from build123d import *

# Parameters (mm, degrees)
SKETCH1_W           = 60
SKETCH1_H           = 80
BOSS_EXTRUDE1_DEPTH = 4
SKETCH2_R           = 1.25
CUT_EXTRUDE1_DEPTH  = 51.159744816
BOSS_EXTRUDE2_START = 2
SKETCH3_R           = 3
SKETCH3_R_2         = 1.25
BOSS_EXTRUDE2_DEPTH = 2
SKETCH4_R           = 1.25
CUT_EXTRUDE2_DEPTH  = 51.358713248
BOSS_EXTRUDE3_START = 2
SKETCH5_R           = 3
SKETCH5_R_2         = 1.25
BOSS_EXTRUDE3_DEPTH = 2
SKETCH7_W           = 12.5
SKETCH7_H           = 12.5
CUT_EXTRUDE4_DEPTH  = 4
FILLET3_R           = 1
FILLET2_R           = 3
SKETCH8_W           = 60
SKETCH8_H           = 9
BOSS_EXTRUDE4_DEPTH = 7
CHAMFER1_SIZE       = 2
SKETCH9_R           = 1.45
CUT_EXTRUDE5_DEPTH  = 8


with BuildPart() as part:
    # Sketch1 → Boss-Extrude1 (new body)
    with BuildSketch(Plane.XY):
        Rectangle(SKETCH1_W, SKETCH1_H)
    extrude(amount=BOSS_EXTRUDE1_DEPTH)

    # Sketch2 → Cut-Extrude1 (cut, through all)
    with BuildSketch(Plane.XY.offset(4)):
        with Locations((-24.5, 25)):
            Circle(SKETCH2_R)
        with Locations(Location((24.5, 25, 0), (0, 0, 180))):
            Circle(SKETCH2_R)
        with Locations((24.5, -33)):
            Circle(SKETCH2_R)
        with Locations(Location((-24.5, -33, 0), (0, 0, 180))):
            Circle(SKETCH2_R)
    extrude(amount=-CUT_EXTRUDE1_DEPTH, mode=Mode.SUBTRACT)

    # Sketch3 → Boss-Extrude2 (add)
    # profile 1 of 4: a face of its own
    with BuildSketch(Plane.XY.offset(4).offset(BOSS_EXTRUDE2_START)):
        with Locations((-24.5, 25)):
            Circle(SKETCH3_R)
        with Locations((-24.5, 25)):
            Circle(SKETCH3_R_2, mode=Mode.SUBTRACT)
    # profile 2 of 4: a face of its own
    with BuildSketch(Plane.XY.offset(4).offset(BOSS_EXTRUDE2_START)):
        with Locations((24.5, 25)):
            Circle(SKETCH3_R)
        with Locations((24.5, 25)):
            Circle(SKETCH3_R_2, mode=Mode.SUBTRACT)
    # profile 3 of 4: a face of its own
    with BuildSketch(Plane.XY.offset(4).offset(BOSS_EXTRUDE2_START)):
        with Locations((24.5, -33)):
            Circle(SKETCH3_R)
        with Locations((24.5, -33)):
            Circle(SKETCH3_R_2, mode=Mode.SUBTRACT)
    # profile 4 of 4: a face of its own
    with BuildSketch(Plane.XY.offset(4).offset(BOSS_EXTRUDE2_START)):
        with Locations((-24.5, -33)):
            Circle(SKETCH3_R)
        with Locations((-24.5, -33)):
            Circle(SKETCH3_R_2, mode=Mode.SUBTRACT)
    extrude(amount=-BOSS_EXTRUDE2_DEPTH)

    # Sketch4 → Cut-Extrude2 (cut, through all)
    with BuildSketch(Plane(origin=(0, 0, 0), x_dir=(-1, 0, 0), z_dir=(0, 0, -1))):
        with Locations((-18.772703202, -17.1)):
            Circle(SKETCH4_R)
        with Locations((9.127296798, -17.1)):
            Circle(SKETCH4_R)
        with Locations((-23.872703202, 35)):
            Circle(SKETCH4_R)
        with Locations((24.327296798, 33.7)):
            Circle(SKETCH4_R)
    extrude(amount=-CUT_EXTRUDE2_DEPTH, mode=Mode.SUBTRACT)

    # Sketch5 → Boss-Extrude3 (add)
    # profile 1 of 4: a face of its own
    with BuildSketch(Plane(origin=(0, 0, 0), x_dir=(-1, 0, 0), z_dir=(0, 0, -1)).offset(BOSS_EXTRUDE3_START)):
        with Locations(Location((-23.872703202, 35, 0), (0, 0, 180))):
            Circle(SKETCH5_R)
        with Locations((-23.872703202, 35)):
            Circle(SKETCH5_R_2, mode=Mode.SUBTRACT)
    # profile 2 of 4: a face of its own
    with BuildSketch(Plane(origin=(0, 0, 0), x_dir=(-1, 0, 0), z_dir=(0, 0, -1)).offset(BOSS_EXTRUDE3_START)):
        with Locations(Location((24.327296798, 33.7, 0), (0, 0, 180))):
            Circle(SKETCH5_R)
        with Locations((24.327296798, 33.7)):
            Circle(SKETCH5_R_2, mode=Mode.SUBTRACT)
    # profile 3 of 4: a face of its own
    with BuildSketch(Plane(origin=(0, 0, 0), x_dir=(-1, 0, 0), z_dir=(0, 0, -1)).offset(BOSS_EXTRUDE3_START)):
        with Locations(Location((9.127296798, -17.1, 0), (0, 0, 180))):
            Circle(SKETCH5_R)
        with Locations((9.127296798, -17.1)):
            Circle(SKETCH5_R_2, mode=Mode.SUBTRACT)
    # profile 4 of 4: a face of its own
    with BuildSketch(Plane(origin=(0, 0, 0), x_dir=(-1, 0, 0), z_dir=(0, 0, -1)).offset(BOSS_EXTRUDE3_START)):
        with Locations(Location((-18.772703202, -17.1, 0), (0, 0, 180))):
            Circle(SKETCH5_R)
        with Locations((-18.772703202, -17.1)):
            Circle(SKETCH5_R_2, mode=Mode.SUBTRACT)
    extrude(amount=-BOSS_EXTRUDE3_DEPTH)

    # Sketch7 → Cut-Extrude4 (cut)
    with BuildSketch(Plane.XY.offset(4)):
        with BuildLine():
            Line((-12.5, 35), (-20.544440734, 35))
            ThreePointArc((-20.544440734, 35), (-21.279248479, 31.109748768), (-25, 29.756971925))
            Line((-25, 29.756971925), (-25, 28.968626967))
            ThreePointArc((-25, 28.968626967), (-21.009991553, 26.954441363), (-21.377501001, 22.5))
            Line((-21.377501001, 22.5), (-12.5, 22.5))
            Line((-12.5, 22.5), (-12.5, 35))
        make_face()
        with Locations((-0.25, 28.75)):
            Rectangle(SKETCH7_W, SKETCH7_H)
        with BuildLine():
            Line((19.872703202, 35), (12, 35))
            Line((12, 35), (12, 22.5))
            Line((12, 22.5), (21.377501001, 22.5))
            ThreePointArc((21.377501001, 22.5), (20.894448725, 26.732050808), (24.5, 29))
            Line((24.5, 29), (24.5, 31.049493864))
            ThreePointArc((24.5, 31.049493864), (21.275511179, 31.957863646), (19.872703202, 35))
        make_face()
        with Locations((-0.25, 10.25)):
            Rectangle(SKETCH7_W, SKETCH7_H)
        with Locations((18.25, 10.25)):
            Rectangle(SKETCH7_W, SKETCH7_H)
        with BuildLine():
            Line((6, -2), (-6.5, -2))
            Line((-6.5, -2), (-6.5, -14.083825016))
            ThreePointArc((-6.5, -14.083825016), (-6.286149505, -14.284350509), (-6.087559968, -14.5))
            Line((-6.087559968, -14.5), (6, -14.5))
            Line((6, -14.5), (6, -2))
        make_face()
        with BuildLine():
            Line((24.5, -2), (12, -2))
            Line((12, -2), (12, -14.5))
            Line((12, -14.5), (15.732966371, -14.5))
            ThreePointArc((15.732966371, -14.5), (18.772703202, -13.1), (21.812440032, -14.5))
            Line((21.812440032, -14.5), (24.5, -14.5))
            Line((24.5, -14.5), (24.5, -2))
        make_face()
        with BuildLine():
            ThreePointArc((20.879833952, -20.5), (18.772703202, -21.1), (16.665572451, -20.5))
            Line((16.665572451, -20.5), (12, -20.5))
            Line((12, -20.5), (12, -33))
            Line((12, -33), (20.5, -33))
            ThreePointArc((20.5, -33), (21.671572875, -30.171572875), (24.5, -29))
            Line((24.5, -29), (24.5, -20.5))
            Line((24.5, -20.5), (20.879833952, -20.5))
        make_face()
        with Locations((-0.25, -26.75)):
            Rectangle(SKETCH7_W, SKETCH7_H)
        with Locations((-18.75, 10.25)):
            Rectangle(SKETCH7_W, SKETCH7_H)
        with Locations((-18.75, -8.25)):
            Rectangle(SKETCH7_W, SKETCH7_H)
        with BuildLine():
            Line((-12.5, -20.5), (-25, -20.5))
            Line((-25, -20.5), (-25, -29.031373033))
            ThreePointArc((-25, -29.031373033), (-21.854248689, -30), (-20.5, -33))
            Line((-20.5, -33), (-12.5, -33))
            Line((-12.5, -33), (-12.5, -20.5))
        make_face()
    extrude(amount=-CUT_EXTRUDE4_DEPTH, mode=Mode.SUBTRACT)

    # Fillet3
    fillet3_edges = [part.edges().sort_by_distance(p)[0] for p in [
        (12, 22.5, 2),
        (12, 35, 2),
        (-6.5, 22.5, 2),
        (-6.5, 35, 2),
        (6, 35, 2),
        (6, 22.5, 2),
        (-12.5, 35, 2),
        (-6.5, -33, 2),
        (-6.5, -20.5, 2),
        (6, -20.5, 2),
        (6, -33, 2),
        (12, -33, 2),
        (12, -20.5, 2),
        (24.5, -20.5, 2),
        (12, -14.5, 2),
        (12, -2, 2),
        (24.5, -2, 2),
        (24.5, -14.5, 2),
        (-6.5, -2, 2),
        (6, -2, 2),
        (6, -14.5, 2),
        (-25, -14.5, 2),
        (-25, -2, 2),
        (-12.5, -2, 2),
        (-12.5, -14.5, 2),
        (-25, 4, 2),
        (-25, 16.5, 2),
        (-12.5, 16.5, 2),
        (-12.5, 4, 2),
        (-6.5, 4, 2),
        (-6.5, 16.5, 2),
        (6, 16.5, 2),
        (6, 4, 2),
        (12, 4, 2),
        (12, 16.5, 2),
        (24.5, 16.5, 2),
        (24.5, 4, 2),
        (-25, -20.5, 2),
        (-12.5, -20.5, 2),
        (-12.5, -33, 2),
    ]]
    fillet(fillet3_edges, radius=FILLET3_R)

    # Fillet2
    fillet2_edges = [part.edges().sort_by_distance(p)[0] for p in [
        (-30, 40, 2),
        (30, 40, 2),
    ]]
    fillet(fillet2_edges, radius=FILLET2_R)

    # Sketch8 → Boss-Extrude4 (add)
    with BuildSketch(Plane.XZ.offset(40)):
        with Locations((0, 2)):
            Rectangle(SKETCH8_W, SKETCH8_H)
    extrude(amount=BOSS_EXTRUDE4_DEPTH)

    # Chamfer1
    chamfer1_edges = [part.edges().sort_by_distance(p)[0] for p in [
        (0, -40, -2.5),
        (0, -40, 6.5),
    ]]
    chamfer(chamfer1_edges, length=CHAMFER1_SIZE)

    # Sketch9 → Cut-Extrude5 (cut)
    with BuildSketch(Plane.XZ.offset(47)):
        with Locations(Location((-22.5, 2, 0), (0, 0, 270))):
            Circle(SKETCH9_R)
        with Locations(Location((22.5, 2, 0), (0, 0, 90))):
            Circle(SKETCH9_R)
    extrude(amount=-CUT_EXTRUDE5_DEPTH, mode=Mode.SUBTRACT)


solid = part.part
Verification items for the finished model (mm, model axes). A direction names the side the tool comes from. Coordinates: 2 decimals unless noted, no trailing zeros. Order: outer loops, then holes, each group sorted by start corner. A loop starts at its lowest first (then second) coordinate and runs counter-clockwise, first axis right, second up. Notation, with made-up numbers: (-8.75, -5.75) -> (6.25, -5.75) arc R29 cw to (6.25, 22.25) -> close; hole circle Ø11 at (77, 42). An arc over 180 degrees is marked (long way). Use CSV: the item, a comma, the result in double quotes. Start each with the question number.
Q1. Section check A-A, the plane y = -12. Record the cut outline in (x, z), and give its area (3 significant figures).
Q2. Section check B-B, the plane x = 4. Record the cut outline in (y, z), and give its area (3 significant figures).
Q3. Tool access check on faces 4 (the cylindrical face through (21.5, -32.9, 5)), 5 (the flat face through (20, -16, -2)), 6 (the flat face through (12, 29, 2)). Record the directions out of +Z, -Z, +X, -X, +Y, -Y that give a thin tool (end or side, any length) a straight path to the whole face; none if there is none.
Q4. Thickness scan on line 1 along Y through (x, z) = (5, 3); line 2 along X through (y, z) = (-24, 2.75); line 3 along X through (y, z) = (-42, 2). Record the ranges inside material, lowest first.
Q5. Section check C-C, the plane z = 2. Give the number of separate pieces and of enclosed holes in the cut face, and give its area (3 significant figures).
Q6. Section check D-D, the plane y = 19.5. Record the cut outline in (x, z).
Q7. Depth check by flat-ended pin: P1, Ø1, axis at x = -20.5, y = 17, coming from the -Z side; P2, Ø1.5, axis at x = 16.5, z = 5.5, coming from the +Y side; P3, Ø3, axis at x = 23.87, y = 35, coming from the -Z side; P4, Ø2, axis at x = 24.5, y = -33, coming from the -Z side. Enter the tip coordinate at first touch or a pass-through.
Q8. Draft check along X on faces 1 (the cylindrical face through (-29.14, 39.1, 2.03)), 2 (the flat face through (-0.4, -41, 5.5)), 3 (the cylindrical face through (-21.04, 27.01, 2.03)). Enter one of: +X half, -X half, draft (parallel to the pull), parting line (faces both ways), or undercut.
Returned:
1,outline,"(-30, 0) -> (-25, 0) -> (-25, 4) -> (-30, 4) -> close; (-12.5, 0) -> (-6.5, 0) -> (-6.5, 4) -> (-12.5, 4) -> close; (6, 0) -> (12, 0) -> (12, 4) -> (6, 4) -> close; (24.5, 0) -> (30, 0) -> (30, 4) -> (24.5, 4) -> close"
1,area,"90.0 mm^2"
2,outline,"(-47, -2.5) -> (-42, -2.5) -> (-40, -0.5) -> (-40, 0) -> (-33, 0) -> (-33, 4) -> (-40, 4) -> (-40, 4.5) -> (-42, 6.5) -> (-47, 6.5) -> close; (-20.5, 0) -> (-14.5, 0) -> (-14.5, 4) -> (-20.5, 4) -> close; (-2, 0) -> (4, 0) -> (4, 4) -> (-2, 4) -> close; (16.5, 0) -> (22.5, 0) -> (22.5, 4) -> (16.5, 4) -> close; (35, 0) -> (40, 0) -> (40, 4) -> (35, 4) -> close"
2,area,"179 mm^2"
3,face 4,"+Z"
3,face 5,"-Z, +X, -X, +Y"
3,face 6,"+Z, -Z"
4,line 1,"y = -47 to -33, -20.5 to -14.5, -2 to 4, 16.5 to 22.5, 35 to 40"
4,line 2,"x = -30 to -25, -12.5 to -6.5, 6 to 12, 24.5 to 30"
4,line 3,"x = -30 to -23.95, -21.05 to 21.05, 23.95 to 30"
5,separate pieces,"1"
5,enclosed holes,"20"
5,area,"3,380 mm^2"
6,outline,"(-30, 0) -> (30, 0) -> (30, 4) -> (-30, 4) -> close"
7,P1,"stops at z = 0"
7,P2,"stops at y = -40.25"
7,P3,"stops at z = -2"
7,P4,"passes through"
8,face 1,"-X half"
8,face 2,"draft"
8,face 3,"undercut"
